Here's how the part is built. I have some questions about the finished solid (model axes, mm). Give positions to 0.01 mm unless a question says otherwise; leave off trailing zeros. Write each loop counter-clockwise with the first axis right and the second up, starting at its lowest first coordinate (ties: lowest second). Pieces come first, ordered by that corner, then holes. Notation, with made-up numbers: (-20.5, 62.5) -> (2.5, 62.5) arc R23 ccw to (2.5, 97.5) -> close; hole circle Ø4 at (16, -24.75). An arc over 180 degrees is marked (long way). Return JSON: item names as keys, results as strings.
Autodesk Inventor part; units mm, degrees
ref_plane "YZ Plane" through (0, 0, 0) normal (1, 0, 0) x (0, 1, 0)
ref_plane "XZ Plane" through (0, 0, 0) normal (0, 1, 0) x (-1, 0, 0)
ref_plane "XY Plane" through (0, 0, 0) normal (0, 0, 1) x (1, 0, 0)
sketch "Szkic1" plane through (0, 0, 0) normal (0, 0, 1) x (1, 0, 0)
  circle A0 centre (0, 0) radius 5.5
  dimension "d0" = 11
extrude "Wyciągnięcie proste1" add sketch "Szkic1" along normal blind 18
sketch "Szkic2" plane through (0, 0, 18) normal (0, 0, 1) x (1, 0, 0)
  circle A0 centre (0, 0) radius 2.6
  dimension "d3" = 5.2
extrude "Wyciągnięcie proste2" cut sketch "Szkic2" against normal blind 9
sketch "Szkic3" plane through (0, 0, 0) normal (0, 0, -1) x (-1, 0, 0)
  circle A0 centre (0, 0) radius 2.4
  dimension "d6" = 4.8
extrude "Wyciągnięcie proste3" cut sketch "Szkic3" against normal blind 9
chamfer "Faza1" distance 0.2 angle 45 4 edges at (-5.5, 0, 18) (-5.5, 0, 0) (2.4, 0, 0) (-2.6, 0, 18)
properties part number "wheel_tube"
1. For pin 1 Ø5.5 at (x, y) = (0.5, 0) entering from +Z; pin 2 Ø1.5 at (x, z) = (4, 6) entering from -Y; pin 3 Ø1 at (x, z) = (-4.5, 12.5) entering from -Y; pin 4 Ø1 at (x, z) = (-1.5, 15) entering from +Y, each with a flat end and sliding along its axis, tell me the tip position at first contact or that it passes through.
Taken from the geometry:
{"pin 1": "stops at z = 18", "pin 2": "stops at y = -4.44", "pin 3": "stops at y = -3.77", "pin 4": "stops at y = 5.41"}
2. Suppose I cut it at A-A, the plane x = 0. List the corners of the cut face in (y, z) for me, and give its area (3 significant figures).
Taken from the geometry:
{"outline": "(-5.5, 0.2) -> (-5.3, 0) -> (-2.6, 0) -> (-2.4, 0.2) -> (-2.4, 9) -> (-2.6, 9) -> (-2.6, 17.8) -> (-2.8, 18) -> (-5.3, 18) -> (-5.5, 17.8) -> close; (2.4, 0.2) -> (2.6, 0) -> (5.3, 0) -> (5.5, 0.2) -> (5.5, 17.8) -> (5.3, 18) -> (2.8, 18) -> (2.6, 17.8) -> (2.6, 9) -> (2.4, 9) -> close", "area": "108 mm²"}
3. If we mould it in two halves opening along X, with no side actions, what happens to faces 1 (the face through (-1.29, 2.024, 4.538)), 2 (the face through (2.3, -2.3, 18)), 3 (the face through (-1.19, 5.37, 8.88)), 4 (the face through (-0.338, 2.578, 13.462))? For each: released by +X, released by -X, zero draft, split by the parting line, or undercut.
Taken from the geometry:
{"face 1": "undercut", "face 2": "zero draft", "face 3": "split by the parting line", "face 4": "undercut"}
4. Suppose I cut it at D-D, the plane z = 16. List the corners of the cut face in (x, y) for me, and give its area (3 significant figures).
Taken from the geometry:
{"outline": "circle Ø11 at (0, 0); hole circle Ø5.2 at (0, 0)", "area": "73.8 mm²"}
5. If I drill on line 1 (Y direction, x = 0, z = 7.25); line 2 (Y direction, x = 0, z = 11); line 3 (X direction, y = -1.25, z = 15.5), over which ranges is the centre line in solid material (lowest first)? Write a range as [from, to].
Taken from the geometry:
{"line 1": "y = [-5.5, -2.4], [2.4, 5.5]", "line 2": "y = [-5.5, -2.6], [2.6, 5.5]", "line 3": "x = [-5.36, -2.28], [2.28, 5.36]"}
6. Suppose I cut it at C-C, the plane z = 3.75. List the corners of the cut face in (x, y) for me, and give its area (3 significant figures).
Taken from the geometry:
{"outline": "circle Ø11 at (0, 0); hole circle Ø4.8 at (0, 0)", "area": "76.9 mm²"}
